Verification items for this drawing (mm, ordinates from the low corner). A direction names the side the tool comes from. Round coordinates to 2 decimals unless told otherwise and drop trailing zeros. Write each loop counter-clockwise with the first axis right and the second up, starting at its lowest first coordinate (ties: lowest second). Pieces come first, ordered by that corner, then holes. Notation, with made-up numbers: (18, 72) -> (77, 72) arc R12 cw to (77, 77) -> close; hole circle Ø5 at (16.5, 3). An arc over 180 degrees is marked (long way). Put each result on its own line as item: value. Start each with the question number.
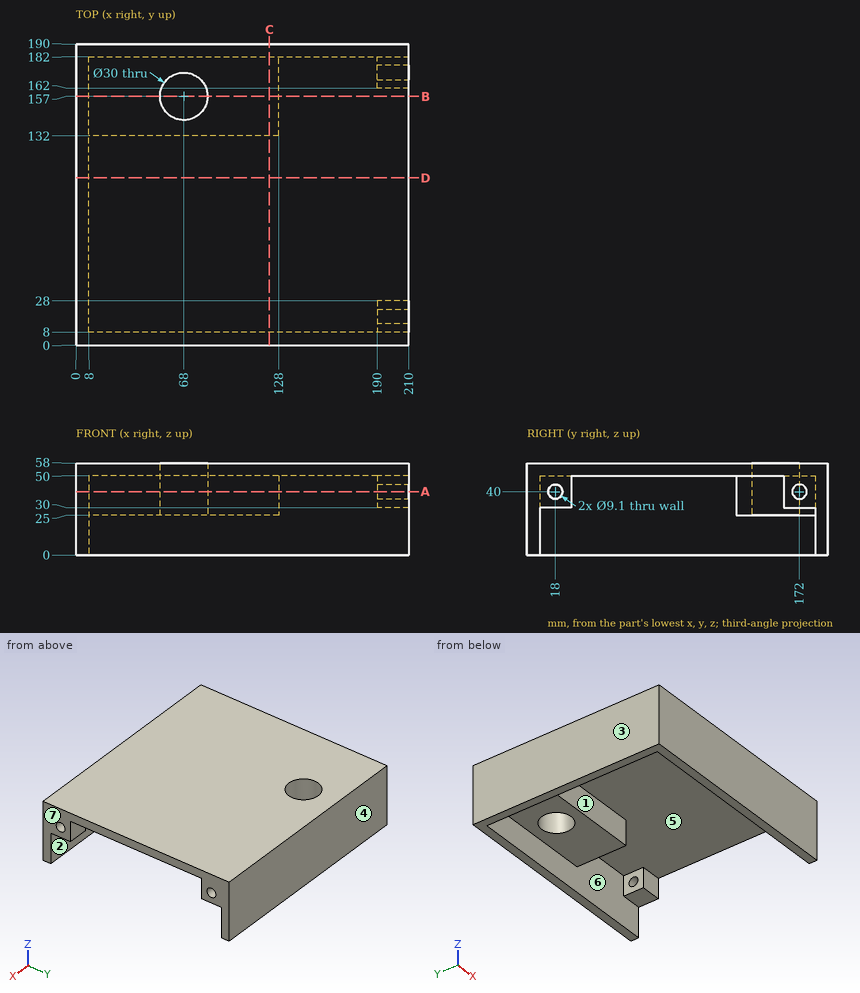
1. Material ranges on L1, parallel to Y at x = 68, z = 41; L2, parallel to Z at x = 196, y = 172; L3, parallel to Y at x = 167, z = 30, recorded low to high. Write a range as [from, to].
2. Access from +Z, -Z, +X, -X, +Y, -Y to the whole of each face (thin tool, end or side, straight path). Record for the marked faces 1, 2 and 3.
3. Section check A-A, the plane z = 40. Enter the section's corners in (x, y), then the cut area to 3 significant figures.
4. Gauge pin test, flat ends, axial feed: P1, Ø5, axis at x = 81.5, y = 143.5, coming from the -Z side; P2, Ø25, axis at y = 91, z = 21.5, coming from the +X side; P3, Ø10, axis at y = 148, z = 26.5, coming from the +X side. Record the tip position at first contact, or that the pin passes through.
5. Draft check along Y on the marked faces 4, 5, 6 and 7. Enter one of: released by +Y, released by -Y, zero draft, split by the parting line, or undercut.
6. Section check C-C, the plane x = 122. Enter the section's corners in (y, z), then the cut area to 3 significant figures.
7. Section check B-B, the plane y = 157. Enter the section's corners in (x, z), then the cut area to 3 significant figures.
8. Section check D-D, the plane y = 105.5. Enter the section's corners in (x, z), then the cut area to 3 significant figures.
Reply:
1. L1: y = [0, 8], [132, 142], [172, 190]
1. L2: z = [30, 35.45], [44.55, 58]
1. L3: y = [0, 8], [182, 190]
2. face 1: -Z, +X
2. face 2: -Z
2. face 3: +Z, -Z, -X, +Y, -Y
3. outline: (0, 0) -> (210, 0) -> (210, 13.45) -> (190, 13.45) -> (190, 8) -> (8, 8) -> (8, 132) -> (128, 132) -> (128, 182) -> (190, 182) -> (190, 176.55) -> (210, 176.55) -> (210, 190) -> (0, 190) -> close; (190, 22.55) -> (210, 22.55) -> (210, 28) -> (190, 28) -> close; (190, 162) -> (210, 162) -> (210, 167.45) -> (190, 167.45) -> close; hole circle Ø30 at (68, 157)
3. area: 10,500 mm2
4. P1: stops at z = 25
4. P2: stops at x = 8
4. P3: stops at x = 128
5. face 4: released by +Y
5. face 5: undercut
5. face 6: undercut
5. face 7: zero draft
6. outline: (0, 0) -> (8, 0) -> (8, 50) -> (132, 50) -> (132, 25) -> (182, 25) -> (182, 0) -> (190, 0) -> (190, 58) -> (0, 58) -> close
6. area: 3,570 mm2
7. outline: (0, 0) -> (8, 0) -> (8, 25) -> (53, 25) -> (53, 58) -> (0, 58) -> close; (83, 25) -> (128, 25) -> (128, 50) -> (210, 50) -> (210, 58) -> (83, 58) -> close
7. area: 4,090 mm2
8. outline: (0, 0) -> (8, 0) -> (8, 50) -> (210, 50) -> (210, 58) -> (0, 58) -> close
8. area: 2,080 mm2
